Verification items for the finished model (mm, model axes). A direction names the side the tool comes from. Coordinates: 2 decimals unless noted, no trailing zeros. Order: outer loops, then holes, each group sorted by start corner. A loop starts at its lowest first (then second) coordinate and runs counter-clockwise, first axis right, second up. Notation, with made-up numbers: (21.5, -35.75) -> (59.5, -35.75) arc R19 cw to (59.5, -13.75) -> close; hole circle Ø2 at (36, 57.25). An arc over 180 degrees is marked (long way). Write item = value, one per line. Start each with the question number.
1. Go/stop test with flat-tipped pins: P1, Ø4, axis at x = -25.4, z = -19.05, coming from the -Y side; P2, Ø12, axis at x = -30, y = 51, coming from the +Z side; P3, Ø4.5, axis at x = 25.4, z = -19.05, coming from the -Y side. Record where each tip stops, or that it passes through.
2. Set-up check for faces 1 (the flat face through (1, 34, -38.1)), 2 (the cylindrical face through (26.578, 11.59, -16.785)), 3 (the conical face through (25.33, 49.95, -23.68)): record each of +Z, -Z, +X, -X, +Y, -Y from which the full face is reachable in a straight line by a thin tool's end or side.
3. Cross-section at A-A on x = -32. Record the cut outline in (y, z), plus the area to 3 significant figures.
4. Cross-section at B-B on z = -30. Record the cut outline in (x, y), plus the area to 3 significant figures.
5. Release check for a two-part mould opening along Y. For faces 4 (the conical face through (-25.47, 49.95, -23.68)), 5 (the flat face through (1, 0, -19)), 6 (the cylindrical face through (-27.43, 11.59, -17.5)) record: +Y half, -Y half, draft (parallel to the pull), parting line (faces both ways), or undercut.
6. Thickness scan on line 1 along X through (y, z) = (6, -19.05); line 2 along Z through (x, y) = (25.4, 6.5); line 3 along Y through (x, z) = (-31.5, -23). Record the ranges inside material, lowest first. Write a range as from..to.
from build123d import *

# Parameters (mm, degrees)
BOSS_EXTRUDE2_DEPTH         = 39.6875
F_1_4_20_TAPPED_HOLE1_D     = 5.1054
F_1_4_20_TAPPED_HOLE1_DEPTH = 22.86
F_1_4_20_TAPPED_HOLE1_TIP   = 1.533816902
F_8_32_TAPPED_HOLE1_D       = 3.4544
F_8_32_TAPPED_HOLE1_DEPTH   = 14.986
F_8_32_TAPPED_HOLE1_TIP     = 1.037806461


with BuildPart() as part:
    # Sketch3 → Boss-Extrude2 (new, symmetric)
    with BuildSketch(Plane(origin=(0, 0, 0), x_dir=(0, 0, -1), z_dir=(1, 0, 0))):
        Polygon((0, 0), (38.1, 0), (38.1, 68.58), (0, 61.861942035), align=None)
    extrude(amount=BOSS_EXTRUDE2_DEPTH, both=True)

    # 1/4-20 Tapped Hole1
    with Locations(Plane(origin=(0, 0, 0), x_dir=(-1, 0, 0), z_dir=(0, -1, 0))):
        with Locations((25.4, 19.05), (-25.4, 19.05)):
            Hole(F_1_4_20_TAPPED_HOLE1_D / 2, depth=F_1_4_20_TAPPED_HOLE1_DEPTH)
            with Locations((0, 0, -(F_1_4_20_TAPPED_HOLE1_DEPTH + F_1_4_20_TAPPED_HOLE1_TIP / 2))):  # 118° drill point
                Cone(0, F_1_4_20_TAPPED_HOLE1_D / 2, F_1_4_20_TAPPED_HOLE1_TIP, mode=Mode.SUBTRACT)

    # #8-32 Tapped Hole1
    with Locations(Plane(origin=(0, 59.996576236, 10.579015141), x_dir=(1, 0, 0), z_dir=(0, 0.9848077530122092, 0.17364817766692348))):
        with Locations((-25.4, 32.284967414), (25.4, 32.284967414)):
            Hole(F_8_32_TAPPED_HOLE1_D / 2, depth=F_8_32_TAPPED_HOLE1_DEPTH)
            with Locations((0, 0, -(F_8_32_TAPPED_HOLE1_DEPTH + F_8_32_TAPPED_HOLE1_TIP / 2))):  # 118° drill point
                Cone(0, F_8_32_TAPPED_HOLE1_D / 2, F_8_32_TAPPED_HOLE1_TIP, mode=Mode.SUBTRACT)


solid = part.part
Worked out:
q1.P1 = 23.19
q1.P2 = 0
q1.P3 = 23.04
q2.face_1 = -Z, +X, -X, +Y, -Y
q2.face_2 = -Y
q2.face_3 = none
q3.outline = (0, -38.1) -> (68.58, -38.1) -> (61.86, 0) -> (0, 0) -> close
q3.area = 2,480 mm²
q4.outline = (-39.69, 0) -> (39.69, 0) -> (39.69, 67.15) -> (-39.69, 67.15) -> close
q4.area = 5,330 mm²
q5.face_4 = undercut
q5.face_5 = -Y half
q5.face_6 = draft
q6.line_1 = -39.69..-27.95, -22.85..22.85, 27.95..39.69
q6.line_2 = -38.1..-21.6, -16.5..0
q6.line_3 = 0..65.92
